Part model, mm, in its own coordinate system. Face numbers are marked on the shaded views. A direction names the side the tool comes from. Coordinates: 2 decimals unless noted, no trailing zeros. Loops run counter-clockwise (first coordinate to the right, second up) from the corner with the lowest first, then second, coordinate; pieces in that order, holes last. Notation, with made-up numbers: (29, 47) - (61, 47) arc R16 ccw to (61, 67) - close; hole circle Ø6 at (16, 55.5). An arc over 180 degrees is marked (long way). One line per question, with ' | ' between items. Start each with the question number.
from build123d import *

# Parameters (mm, degrees)
SKETCH1_W                = 1
SKETCH1_H                = 6
BOSS_EXTRUDE1_DEPTH      = 3
BOSS_EXTRUDE1_DEPTH_BACK = 3
SKETCH9_W                = 6
SKETCH9_H                = 1.15698482
FILLET1_R                = 2


with BuildPart() as part:
    # Sketch1 → Revolve3 (revolve)
    with BuildSketch(Plane.XY, mode=Mode.PRIVATE) as revolve3_sk:
        Rectangle(SKETCH1_W, SKETCH1_H)
    revolve(revolve3_sk.sketch.rotate(Axis((-0.5, -3, 0), (0, 1, 0)), 90), axis=Axis((-0.5, -3, 0), (0, 1, 0)))

    # Sketch9 → Boss-Extrude1 (add, two sides: drawn at the far end of the back side and taken through both)
    with BuildSketch(Plane.XY.offset(-BOSS_EXTRUDE1_DEPTH_BACK)):
        with Locations((-0.5, 3.57849241)):
            Rectangle(SKETCH9_W, SKETCH9_H)
    extrude(amount=BOSS_EXTRUDE1_DEPTH + BOSS_EXTRUDE1_DEPTH_BACK)

    # Fillet1
    fillet1_edges = [part.edges().sort_by_distance(p)[0] for p in [
        (-3.5, 3.57849241, -3),
        (2.5, 3.57849241, -3),
        (-3.5, 3.57849241, 3),
        (2.5, 3.57849241, 3),
    ]]
    fillet(fillet1_edges, radius=FILLET1_R)


solid = part.part
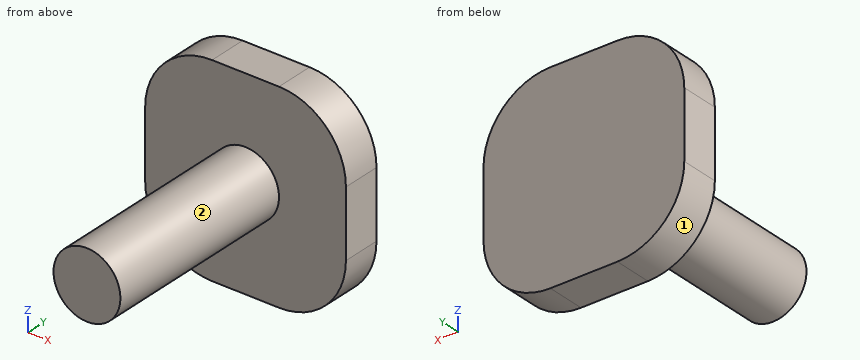
1) Tool access for the marked faces 1 and 2: list every direction of +Z, -Z, +X, -X, +Y, -Y with a clear straight run to the whole face (end or side of a thin tool).
2) Band-saw the part on D-D on x = 2.25. List the corners of the cut face in (y, z), then the cut area to 3 significant figures.
3) Band-saw the part on C-C on y = 2. List the corners of the cut face in (x, z).
4) Band-saw the part on A-A on z = 0. List the corners of the cut face in (x, y), then the cut area to 3 significant figures.
5) Wall check: line 1 along Y through (x, z) = (0.5, 1); line 2 along X through (y, z) = (0.5, 0); line 3 along X through (y, z) = (3.75, 2). Give the ranges that are in metal, low to high. Write a range as [from, to].
6) Pin check, flat tip, straight feed: pin 1 Ø2 at (x, y) = (-1, 0) entering from -Z. Stop position of the tip, or through.
7) Band-saw the part on B-B on x = -0.5. List the corners of the cut face in (y, z), then the cut area to 3 significant figures.
Values found:
1) face 1: -Z, -X, +Y, -Y | face 2: -Y
2) outline: (3, -1.97) - (4.16, -1.97) - (4.16, 1.97) - (3, 1.97) - close | area: 4.55 mm²
3) outline: circle Ø2 at (-0.5, 0)
4) outline: (-3.5, 3) - (-1.5, 3) - (-1.5, -3) - (0.5, -3) - (0.5, 3) - (2.5, 3) - (2.5, 4.16) - (-3.5, 4.16) - close | area: 18.9 mm²
5) line 1: [3, 4.16] | line 2: [-1.5, 0.5] | line 3: [-3.23, 2.23]
6) pin 1: z = -1
7) outline: (-3, -1) - (3, -1) - (3, -3) - (4.16, -3) - (4.16, 3) - (3, 3) - (3, 1) - (-3, 1) - close | area: 18.9 mm²
